Could you check a few things on this drawing? It's one solid part, dimensions in mm from its lowest x, y, z. A direction names the side the tool comes from. Round coordinates to 2 decimals unless told otherwise and drop trailing zeros. Write each loop counter-clockwise with the first axis right and the second up, starting at its lowest first coordinate (ties: lowest second). Pieces come first, ordered by that corner, then holes. Notation, with made-up numbers: M 67.5,56 L 76.5,56 A23 ccw 76.5,93 Z; hole C 37,56 d4. An arc over 180 degrees is marked long. One line per item, written item: value. Start each with the question number.
(1) Which directions (+Z, -Z, +X, -X, +Y, -Y) give clear straight access to the entire face, cutting with the end or side of a thin tool? Please do the marked faces 1 and 2.
(2) I'm going to push flat-ended pins straight in: pin 1 Ø1 at (x, y) = (11, 12) entering from +Z; pin 2 Ø3 at (x, z) = (33, 11.5) entering from +Y; pin 3 Ø2 at (x, z) = (23, 7) entering from +Y. Where does each tip first touch, or does it pass through?
(3) Thinking about a two-plate mould opening in X: for the marked faces 3 and 4, which applies, released by +X, released by -X, zero draft, split by the parting line, or undercut?
(4) I want a section at A-A on z = 23. Please give me the cut outline in (x, y), and give its area (3 significant figures).
(5) If I drill on L1, parallel to X at y = 17.45, z = 31 (1 decimal); L2, parallel to Y at x = 30.5, z = 11.5; L3, parallel to X at y = 18.25, z = 7, over which ranges is the centre line in solid material (lowest first)?
(6) I want a section at B-B on x = 23. Please give me the cut outline in (y, z).
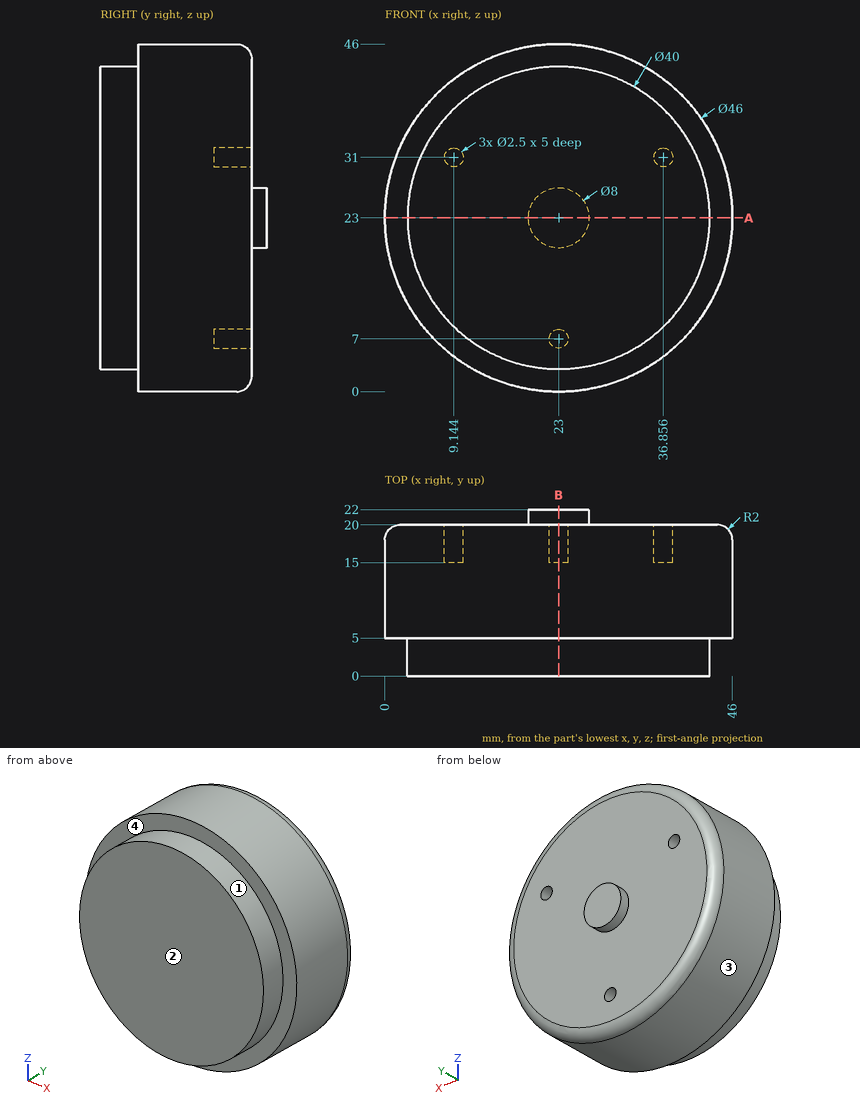
Found:
1. face 1: -Y
1. face 2: +Z, -Z, +X, -X, -Y
2. pin 1: stops at z = 42.92
2. pin 2: stops at y = 20
2. pin 3: stops at y = 15
3. face 3: split by the parting line
3. face 4: zero draft
4. outline: M 0,5 L 3,5 L 3,0 L 43,0 L 43,5 L 46,5 L 46,18 A2 ccw 44,20 L 27,20 L 27,22 L 19,22 L 19,20 L 2,20 A2 ccw 0,18 Z
4. area: 904 mm²
5. L1: x = 1.4 to 7.9, 10.4 to 35.6, 38.1 to 44.6
5. L2: y = 0 to 20
5. L3: x = 6.5 to 21.75, 24.25 to 39.5
6. outline: M 0,3 L 5,3 L 5,0 L 18,0 A2 ccw 20,2 L 20,5.75 L 15,5.75 L 15,8.25 L 20,8.25 L 20,19 L 22,19 L 22,27 L 20,27 L 20,44 A2 ccw 18,46 L 5,46 L 5,43 L 0,43 Z
